Read the model definition and answer for the solid it produces. Units are mm, in the model's axes. A direction names the side the tool comes from. Round coordinates to 2 decimals unless told otherwise and drop trailing zeros. Order: outer loops, then holes, each group sorted by start corner. A loop starts at its lowest first (then second) coordinate and runs counter-clockwise, first axis right, second up. Notation, with made-up numbers: (34.5, 64.25) - (86.5, 64.25) arc R33 ccw to (86.5, 97.25) - close; hole circle Ø7 at (-31, 19). An arc over 180 degrees is marked (long way). Put each result on its own line as item: value. Start each with the question number.
Q1. Section A-A on x = 0 is taken. Give the vertices of the cut face in (y, z), then the cut area to 3 significant figures.
Q2. Section C-C on z = -5.25 is taken. Give the vertices of the cut face in (x, y).
Q3. Section D-D on x = -5 is taken. Give the vertices of the cut face in (y, z) (3 decimals), then the cut area to 3 significant figures.
Q4. Which of the six approach directions +Z, -Z, +X, -X, +Y, -Y give full straight-line access (tool end or side, diameter ignored) to faces 4 (the face through (0, 3, -6)), 5 (the face through (0, 5.5, -1))?
Q5. Find the intervals of material crossed by line 1 along Y through (x, z) = (0, 0); line 2 along X through (y, z) = (-7.75, -3.75); line 3 along Y through (x, z) = (-3, -1.5), in increasing order. Write a range as from..to.
Q6. For a pull along X with two mould halves and no side action, classify faces 1 (the face through (0, -12, -6)), 2 (the face through (-3.695, -6.032, -2.741)), 3 (the face through (0, -14.5, -1)) as pulls with the +X half, pulls with the -X half, needs draft (parallel to the pull), parting line crosses it, or undercut.
Q7. Section B-B on y = -8 is taken. Give the vertices of the cut face in (x, z).
Q8. This flat-tipped pin is pushed along its axis until it touches: pin 1 Ø1 at (x, y) = (-0.5, 3) entering from -Z. Where does it stop, or does it pass through?
from build123d import *

# Parameters (mm, degrees)
F1_DEPTH = 9
F3_D     = 8
F5_DEPTH = 5.5
F7_DEPTH = 5.5


with BuildPart() as f1:
    # F0 (on Front) → F1 (new body)
    with BuildSketch(Plane.XZ):
        with BuildLine():
            ThreePointArc((-7.542472, 2.666667), (-7.884788, 1.352816), (-8, 0))
            ThreePointArc((-8, 0), (1.352816, -7.884788), (7.542472, 2.666667))
            Line((7.542472, 2.666667), (-7.542472, 2.666667))
        make_face()
    extrude(amount=F1_DEPTH)

    # F3 (through all)
    with Locations(Plane.XY.offset(2.666667)):
        with Locations((0, -4.5)):
            Hole(F3_D / 2)

    # F4 (on face) → F5 (join)
    with BuildSketch(Plane.XZ.offset(9)):
        with BuildLine():
            Line((5.374838, 2.666667), (-5.374838, 2.666667))
            ThreePointArc((-5.374838, 2.666667), (0, -6), (5.374838, 2.666667))
        make_face()
    extrude(amount=F5_DEPTH)

    # F6 (on face) → F7 (join)
    with BuildSketch(Plane(origin=(0, 0, 0), x_dir=(-1, 0, 0), z_dir=(0, 1, 0))):
        with BuildLine():
            Line((5.374838, 2.666667), (-5.374838, 2.666667))
            ThreePointArc((-5.374838, 2.666667), (0, -6), (5.374838, 2.666667))
        make_face()
    extrude(amount=F7_DEPTH)


solid = f1.part
Findings:
1. outline: (-14.5, -6) - (-9, -6) - (-9, -8) - (-8.5, -8) - (-8.5, 2.67) - (-14.5, 2.67) - close; (-0.5, -8) - (0, -8) - (0, -6) - (5.5, -6) - (5.5, 2.67) - (-0.5, 2.67) - close
1. area: 106 mm2
2. outline: (-6.04, -9) - (-2.9, -9) - (-2.9, -14.5) - (2.9, -14.5) - (2.9, -9) - (6.04, -9) - (6.04, 0) - (2.9, 0) - (2.9, 5.5) - (-2.9, 5.5) - (-2.9, 0) - (-6.04, 0) - close; hole circle Ø8 at (0, -4.5)
3. outline: (-14.5, -3.317) - (-9, -3.317) - (-9, -6.245) - (0, -6.245) - (0, -3.317) - (5.5, -3.317) - (5.5, 2.667) - (-14.5, 2.667) - close
3. area: 146 mm2
4. face 4: +Y
4. face 5: +Z, -Z, +X, -X, +Y
5. line 1: -14.5..-8.5, -0.5..5.5
5. line 2: -7.07..-2.33, 2.33..7.07
5. line 3: -14.5..-7.15, -1.85..5.5
6. face 1: parting line crosses it
6. face 2: undercut
6. face 3: needs draft
7. outline: (-8, 0) arc R8 ccw to (-1.94, -7.76) - (-1.94, 2.67) - (-7.54, 2.67) arc R8 ccw to start; (1.94, -7.76) arc R8 ccw to (7.54, 2.67) - (1.94, 2.67) - close
8. pin 1: z = -6
